Verification items for the finished model (mm, model axes). Give positions to 0.01 mm unless a question says otherwise; leave off trailing zeros. Write each loop counter-clockwise with the first axis right and the second up, starting at its lowest first coordinate (ties: lowest second). Pieces come first, ordered by that corner, then holes. Notation, with made-up numbers: (12, 49) -> (21, 49) arc R11 cw to (21, 62) -> close; hole circle Ø1 at (47, -4). An arc over 180 degrees is marked (long way). Use one line per item in the form item = value. Start each with the question number.
(1) Scan lines: L1, parallel to Z at x = 53, y = 2.25; L2, parallel to X at y = 1.95, z = -51; L3, parallel to X at y = 1.1, z = 50.5. Record each from-to range of solid material in increasing order.
(2) Section check A-A, the plane x = -47. Record the cut outline in (y, z), plus the area to 3 significant figures.
(3) Section check C-C, the plane x = 46. Record the cut outline in (y, z).
(4) Section check B-B, the plane y = 1.25. State how many separate pieces and enclosed holes the cut face has, plus the area to 3 significant figures.
(5) Section check D-D, the plane x = -13.5. Record the cut outline in (y, z), plus the area to 3 significant figures.
(6) Depth check by flat-ended pin: pin 1 Ø2 at (x, z) = (-54.95, 51) entering from +Y; pin 2 Ø3 at (x, z) = (-7, -26) entering from -Y; pin 3 Ø1 at (x, y) = (31.5, 0.5) entering from -Z; pin 4 Ø0.6 at (x, y) = (-6.5, 1.5) entering from +Z. Enter the tip coordinate at first touch or a pass-through.
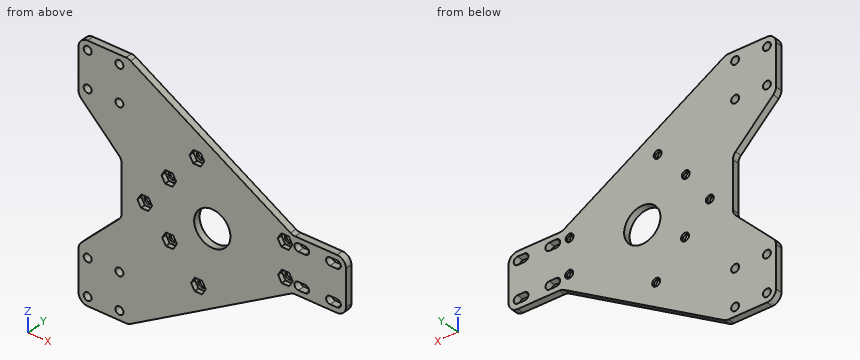
from build123d import *

# Parameters (mm, degrees)
ESQUISSE1_W             = 117.9
ESQUISSE1_H             = 110
BOSS_EXTRU_1_DEPTH      = 3
ESQUISSE2_R             = 1.75
ENL_V_MAT_EXTRU_1_DEPTH = 81.679009042
CONG_1_R                = 4
ESQUISSE3_R             = 8
ENL_V_MAT_EXTRU_2_DEPTH = 81.679009042
ENL_V_MAT_EXTRU_3_DEPTH = 2.1
ESQUISSE19_R            = 1.75
ENL_V_MAT_EXTRU_4_DEPTH = 81.679009042


with BuildPart() as part:
    # Esquisse1 → Boss.-Extru.1 (new body)
    with BuildSketch(Plane(origin=(0, 0, 0), x_dir=(1, 0, 0), z_dir=(0, 1, 0))):
        Rectangle(ESQUISSE1_W, ESQUISSE1_H)
    extrude(amount=BOSS_EXTRU_1_DEPTH)

    # Esquisse2 → Enlèv. mat.-Extru.1 (cut, through all)
    with BuildSketch(Plane(origin=(0, 0, 0), x_dir=(1, 0, 0), z_dir=(0, 1, 0))):
        with Locations(Location((-40.95, -35, 0), (0, 0, 270))):
            Circle(ESQUISSE2_R)
        with Locations(Location((-54.95, -35, 0), (0, 0, 270))):
            Circle(ESQUISSE2_R)
        with Locations(Location((-54.95, -51, 0), (0, 0, 270))):
            Circle(ESQUISSE2_R)
        with Locations(Location((-40.95, -51, 0), (0, 0, 270))):
            Circle(ESQUISSE2_R)
        with Locations(Location((-40.95, 51, 0), (0, 0, 90))):
            Circle(ESQUISSE2_R)
        with Locations(Location((-54.95, 51, 0), (0, 0, 90))):
            Circle(ESQUISSE2_R)
        with Locations(Location((-54.95, 35, 0), (0, 0, 90))):
            Circle(ESQUISSE2_R)
        with Locations(Location((-40.95, 35, 0), (0, 0, 90))):
            Circle(ESQUISSE2_R)
        Polygon((58.95, 12), (35.45, 12), (-36.95, 55), (58.95, 55), align=None)
        Polygon((58.95, -12), (35.45, -12), (-36.95, -55), (58.95, -55), align=None)
        Polygon((-58.95, -31), (-39.95, -12), (-39.95, 12), (-58.95, 31), align=None)
        with BuildLine():
            Line((37.95, 9.75), (40.95, 9.75))
            ThreePointArc((40.95, 9.75), (42.7, 8), (40.95, 6.25))
            Line((40.95, 6.25), (37.95, 6.25))
            ThreePointArc((37.95, 6.25), (36.2, 8), (37.95, 9.75))
        make_face()
        with BuildLine():
            Line((54.95, 6.25), (51.95, 6.25))
            ThreePointArc((51.95, 6.25), (50.2, 8), (51.95, 9.75))
            Line((51.95, 9.75), (54.95, 9.75))
            ThreePointArc((54.95, 9.75), (56.7, 8), (54.95, 6.25))
        make_face()
        with BuildLine():
            Line((37.95, -6.25), (40.95, -6.25))
            ThreePointArc((40.95, -6.25), (42.7, -8), (40.95, -9.75))
            Line((40.95, -9.75), (37.95, -9.75))
            ThreePointArc((37.95, -9.75), (36.2, -8), (37.95, -6.25))
        make_face()
        with BuildLine():
            Line((54.95, -9.75), (51.95, -9.75))
            ThreePointArc((51.95, -9.75), (50.2, -8), (51.95, -6.25))
            Line((51.95, -6.25), (54.95, -6.25))
            ThreePointArc((54.95, -6.25), (56.7, -8), (54.95, -9.75))
        make_face()
    extrude(amount=ENL_V_MAT_EXTRU_1_DEPTH, mode=Mode.SUBTRACT)

    # Congé1
    cong_1_edges = [part.edges().sort_by_distance(p)[0] for p in [
        (-39.95, 1.5, -12),
        (-58.95, 1.5, -55),
        (-58.95, 1.5, 55),
        (58.95, 1.5, 12),
        (35.45, 1.5, 12),
        (-36.95, 1.5, 55),
        (58.95, 1.5, -12),
        (-36.95, 1.5, -55),
        (35.45, 1.5, -12),
        (-58.95, 1.5, -31),
        (-58.95, 1.5, 31),
        (-39.95, 1.5, 12),
    ]]
    fillet(cong_1_edges, radius=CONG_1_R)

    # Esquisse3 → Enlèv. mat.-Extru.2 (cut, through all)
    with BuildSketch(Plane(origin=(0, 0, 0), x_dir=(1, 0, 0), z_dir=(0, 1, 0))):
        with Locations(Location((0, 0, 0), (0, 0, 270))):
            Circle(ESQUISSE3_R)
    extrude(amount=ENL_V_MAT_EXTRU_2_DEPTH, mode=Mode.SUBTRACT)

    # Esquisse6 → Enlèv. mat.-Extru.3 (cut)
    with BuildSketch(Plane.XZ):
        Polygon((-15.609293528, -12.883492858), (-17.225874282, -10.083492858), (-20.45903579, -10.083492858), (-22.075616543, -12.883492858), (-20.45903579, -15.683492858), (-17.225874282, -15.683492858), align=None)
        Polygon((-26.54852785, -1.667626755), (-28.165108604, 1.132373245), (-31.398270112, 1.132373245), (-33.014850865, -1.667626755), (-31.398270112, -4.467626755), (-28.165108604, -4.467626755), align=None)
        Polygon((-15.926426125, 12.814550393), (-17.543006878, 15.614550393), (-20.776168386, 15.614550393), (-22.39274914, 12.814550393), (-20.776168386, 10.014550393), (-17.543006878, 10.014550393), align=None)
        Polygon((-3.541855014, 26.331929262), (-5.158435767, 29.131929262), (-8.391597275, 29.131929262), (-10.008178029, 26.331929262), (-8.391597275, 23.531929262), (-5.158435767, 23.531929262), align=None)
        Polygon((35.306333009, 7.982986542), (33.689752255, 10.782986542), (30.456590748, 10.782986542), (28.840009994, 7.982986542), (30.456590748, 5.182986542), (33.689752255, 5.182986542), align=None)
        Polygon((35.491429855, -7.015871386), (33.874849101, -4.215871386), (30.641687594, -4.215871386), (29.02510684, -7.015871386), (30.641687594, -9.815871386), (33.874849101, -9.815871386), align=None)
        Polygon((-2.892117597, -26.317910049), (-4.508698351, -23.517910049), (-7.741859858, -23.517910049), (-9.358440612, -26.317910049), (-7.741859858, -29.117910049), (-4.508698351, -29.117910049), align=None)
    extrude(amount=-ENL_V_MAT_EXTRU_3_DEPTH, mode=Mode.SUBTRACT)

    # Esquisse19 → Enlèv. mat.-Extru.4 (cut, through all)
    with BuildSketch(Plane.XZ):
        with Locations(Location((-29.781689358, -1.667626755, 0), (0, 0, 270))):
            Circle(ESQUISSE19_R)
        with Locations(Location((-19.159587632, 12.814550393, 0), (0, 0, 270))):
            Circle(ESQUISSE19_R)
        with Locations(Location((-6.775016521, 26.331929262, 0), (0, 0, 270))):
            Circle(ESQUISSE19_R)
        with Locations(Location((-18.842455036, -12.883492858, 0), (0, 0, 270))):
            Circle(ESQUISSE19_R)
        with Locations(Location((-6.125279104, -26.317910049, 0), (0, 0, 270))):
            Circle(ESQUISSE19_R)
        with Locations(Location((32.258268348, -7.015871386, 0), (0, 0, 270))):
            Circle(ESQUISSE19_R)
        with Locations(Location((32.073171502, 7.982986542, 0), (0, 0, 270))):
            Circle(ESQUISSE19_R)
    extrude(amount=-ENL_V_MAT_EXTRU_4_DEPTH, mode=Mode.SUBTRACT)


solid = part.part
Completed:
q1.L1 = -12 to -9.75, -6.25 to 6.25, 9.75 to 12
q1.L2 = -58.95 to -56.7, -53.2 to -42.7, -39.2 to -30.22
q1.L3 = -58.95 to -56.63, -53.27 to -42.63, -39.27 to -29.37
q2.outline = (0, -55) -> (3, -55) -> (3, -19.05) -> (0, -19.05) -> close; (0, 19.05) -> (3, 19.05) -> (3, 55) -> (0, 55) -> close
q2.area = 216 mm²
q3.outline = (0, -12) -> (3, -12) -> (3, 12) -> (0, 12) -> close
q4.separate_pieces = 1
q4.enclosed_holes = 20
q4.area = 6,460 mm²
q5.outline = (0, -41.07) -> (3, -41.07) -> (3, 41.07) -> (0, 41.07) -> close
q5.area = 246 mm²
q6.pin_1 = through
q6.pin_2 = 2.1
q6.pin_3 = -14.64
q6.pin_4 = 37.09
